```python
from build123d import *

# Parameters (mm, degrees)
SKETCH1_R                             = 14
BOSS_EXTRUDE1_DEPTH                   = 4.75
BOSS_EXTRUDE4_DEPTH                   = 7.61416499
BOSS_EXTRUDE5_START                   = 7.61416499
SKETCH5_R                             = 14
BOSS_EXTRUDE5_DEPTH                   = 7.61416499
TAP_DRILL_FOR_M4X0_7_TAP2_D           = 3.3
TAP_DRILL_FOR_M4X0_7_TAP2_DEPTH       = 13.724
TAP_DRILL_FOR_M4X0_7_TAP2_CSINK_D     = 3.35
TAP_DRILL_FOR_M4X0_7_TAP2_CSINK_ANGLE = 90
TAP_DRILL_FOR_M4X0_7_TAP2_TIP         = 0.991420021
FILLET2_R                             = 1
CBORE_FOR_M2_SHCS3_AT_2_COUNT         = 2
CBORE_FOR_M2_SHCS3_AT_2_PITCH         = 6.122934918
CBORE_FOR_M2_SHCS3_AT_3_COUNT         = 2
CBORE_FOR_M2_SHCS3_AT_3_PITCH         = 11.313708499
CBORE_FOR_M2_SHCS3_AT_4_COUNT         = 2
CBORE_FOR_M2_SHCS3_AT_4_PITCH         = 14.78207252
CBORE_FOR_M2_SHCS3_AT_5_COUNT         = 2
CBORE_FOR_M2_SHCS3_AT_5_PITCH         = 16
CBORE_FOR_M2_SHCS3_AT_6_COUNT         = 2
CBORE_FOR_M2_SHCS3_AT_6_PITCH         = 14.78207252
SKETCH20_R                            = 4
CUT_EXTRUDE2_DEPTH                    = 2.75
SKETCH21_R                            = 2
CUT_EXTRUDE3_DEPTH                    = 2.5


with BuildPart() as part:
    # Sketch1 → Boss-Extrude1 (new body)
    with BuildSketch(Plane(origin=(0, 0, 0), x_dir=(1, 0, 0), z_dir=(0, 1, 0))):
        with Locations(Location((0, 0, 0), (0, 0, 270))):
            Circle(SKETCH1_R)
    extrude(amount=-BOSS_EXTRUDE1_DEPTH)

    # Sketch4 → Boss-Extrude4 (add)
    with BuildSketch(Plane(origin=(0, 0, 0), x_dir=(1, 0, 0), z_dir=(0, 1, 0))):
        with BuildLine():
            ThreePointArc((3.9, 0), (3.062596937, 2.414642831), (0.91, 3.792347558))
            Line((0.91, 3.792347558), (-0.91, 3.792347558))
            ThreePointArc((-0.91, 3.792347558), (-2.414642831, -3.062596937), (3.9, 0))
        make_face()
        with BuildLine():
            Line((-0.91, 3.792347558), (0.91, 3.792347558))
            ThreePointArc((0.91, 3.792347558), (0, 3.9), (-0.91, 3.792347558))
        make_face()
        with BuildLine():
            Line((0.91, 3.792347558), (0.91, 4.821959978))
            Line((0.91, 4.821959978), (-0.91, 4.821959978))
            Line((-0.91, 4.821959978), (-0.91, 3.792347558))
            ThreePointArc((-0.91, 3.792347558), (0, 3.9), (0.91, 3.792347558))
        make_face()
    extrude(amount=BOSS_EXTRUDE4_DEPTH)

    # Sketch5 → Boss-Extrude5 (add)
    with BuildSketch(Plane(origin=(0, 0, 0), x_dir=(1, 0, 0), z_dir=(0, 1, 0)).offset(BOSS_EXTRUDE5_START)):
        with Locations(Location((0, 0, 0), (0, 0, 270))):
            Circle(SKETCH5_R)
        with BuildLine():
            ThreePointArc((-6.116473657, 8.411227616), (10.4, 0), (-6.116473657, -8.411227616))
            Line((-6.116473657, -8.411227616), (-6.116473657, -6.116473657))
            ThreePointArc((-6.116473657, -6.116473657), (-8.65, 0), (-6.116473657, 6.116473657))
            Line((-6.116473657, 6.116473657), (-6.116473657, 8.411227616))
        make_face(mode=Mode.SUBTRACT)
    extrude(amount=-BOSS_EXTRUDE5_DEPTH)

    # Tap Drill for M4x0.7 Tap2
    with Locations(Plane(origin=(-20, 0, 0), x_dir=(0, 0, -1), z_dir=(-1, 0, 0))):
        with Locations((0, -4.48916499)):
            CounterSinkHole(TAP_DRILL_FOR_M4X0_7_TAP2_D / 2, TAP_DRILL_FOR_M4X0_7_TAP2_CSINK_D / 2, depth=TAP_DRILL_FOR_M4X0_7_TAP2_DEPTH, counter_sink_angle=TAP_DRILL_FOR_M4X0_7_TAP2_CSINK_ANGLE)
            with Locations((0, 0, -(TAP_DRILL_FOR_M4X0_7_TAP2_DEPTH + TAP_DRILL_FOR_M4X0_7_TAP2_TIP / 2))):  # 118° drill point
                Cone(0, TAP_DRILL_FOR_M4X0_7_TAP2_D / 2, TAP_DRILL_FOR_M4X0_7_TAP2_TIP, mode=Mode.SUBTRACT)

    # Fillet2
    fillet2_edges = [part.edges().sort_by_distance(p)[0] for p in [
        (-6.116473657, 3.807082495, -8.411227616),
        (-6.116473657, 3.807082495, 8.411227616),
        (-6.116473657, 3.807082495, 6.116473657),
        (-6.116473657, 3.807082495, -6.116473657),
    ]]
    fillet(fillet2_edges, radius=FILLET2_R)

    # Sketch19 → CBORE for M2 SHCS3 (revolve, cut)
    with BuildSketch(Plane(origin=(-3.061467459, 0, -7.39103626), x_dir=(0, 0, 1), z_dir=(1, 0, 0))):
        Polygon((0, 0), (0, 5.471032743), (1.2, 4.75), (1.2, 3.5), (2.2, 3.5), (2.2, 0.025), (2.225, 0), align=None)
    cbore_for_m2_shcs3 = revolve(axis=Axis((-3.061467459, 6.35, -7.39103626), (0, -1, 0)), mode=Mode.SUBTRACT)

    # CBORE for M2 SHCS3 at 2: CBORE for M2 SHCS3 ×2
    with Locations(*[(i * CBORE_FOR_M2_SHCS3_AT_2_PITCH, 0, 0) for i in range(1, CBORE_FOR_M2_SHCS3_AT_2_COUNT)]):
        add(cbore_for_m2_shcs3, mode=Mode.SUBTRACT)

    # CBORE for M2 SHCS3 at 3: CBORE for M2 SHCS3 ×2
    with Locations(*[Vector(0.9238795325112845, 0, 0.38268343236509533) * (i * CBORE_FOR_M2_SHCS3_AT_3_PITCH) for i in range(1, CBORE_FOR_M2_SHCS3_AT_3_COUNT)]):
        add(cbore_for_m2_shcs3, mode=Mode.SUBTRACT)

    # CBORE for M2 SHCS3 at 4: CBORE for M2 SHCS3 ×2
    with Locations(*[Vector(0.7071067811865439, 0, 0.7071067811865512) * (i * CBORE_FOR_M2_SHCS3_AT_4_PITCH) for i in range(1, CBORE_FOR_M2_SHCS3_AT_4_COUNT)]):
        add(cbore_for_m2_shcs3, mode=Mode.SUBTRACT)

    # CBORE for M2 SHCS3 at 5: CBORE for M2 SHCS3 ×2
    with Locations(*[Vector(0.3826834323650841, 0, 0.9238795325112892) * (i * CBORE_FOR_M2_SHCS3_AT_5_PITCH) for i in range(1, CBORE_FOR_M2_SHCS3_AT_5_COUNT)]):
        add(cbore_for_m2_shcs3, mode=Mode.SUBTRACT)

    # CBORE for M2 SHCS3 at 6: CBORE for M2 SHCS3 ×2
    with Locations(*[(0, 0, i * CBORE_FOR_M2_SHCS3_AT_6_PITCH) for i in range(1, CBORE_FOR_M2_SHCS3_AT_6_COUNT)]):
        add(cbore_for_m2_shcs3, mode=Mode.SUBTRACT)

    # Sketch20 → Cut-Extrude2 (cut)
    with BuildSketch(Plane.XZ.offset(4.75)):
        with Locations(Location((0, 0, 0), (0, 0, 270))):
            Circle(SKETCH20_R)
    extrude(amount=-CUT_EXTRUDE2_DEPTH, mode=Mode.SUBTRACT)

    # Sketch21 → Cut-Extrude3 (cut)
    with BuildSketch(Plane(origin=(0, -2, 0), x_dir=(-1, 0, 0), z_dir=(0, -1, 0))):
        with Locations(Location((0, 0, 0), (0, 0, 90))):
            Circle(SKETCH21_R)
    extrude(amount=-CUT_EXTRUDE3_DEPTH, mode=Mode.SUBTRACT)


solid = part.part
```
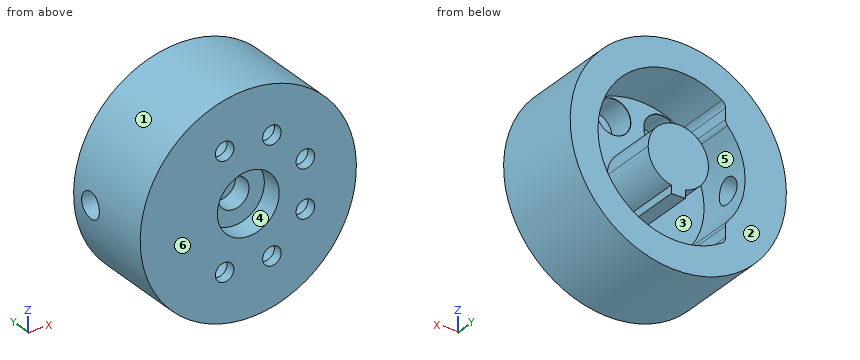
Can you work these out from the model? Positions are in its coordinate system, mm. Face numbers are marked on the shaded views. A direction names the side the tool comes from. Coordinates: 2 decimals unless noted, no trailing zeros. Write each loop counter-clockwise with the first axis right and the second up, starting at its lowest first coordinate (ties: lowest second). Pieces come first, ordered by that corner, then holes. Notation, with made-up numbers: (86.5, -35) - (101.5, -35) arc R26 cw to (101.5, -15) - close; hole circle Ø6 at (35, 14.25). An arc over 180 degrees is marked (long way). Return JSON: item names as keys, results as strings.
Q1. If we section it at B-B (z = 0.5): Please give me the cut outline in (x, y).
Computed values:
{"outline": "(-13.99, -4.75) - (-3.97, -4.75) - (-3.97, -2) - (-1.94, -2) - (-1.94, 0.5) - (1.94, 0.5) - (1.94, -2) - (3.97, -2) - (3.97, -4.75) - (13.99, -4.75) - (13.99, 7.61) - (10.39, 7.61) - (10.39, 0) - (3.87, 0) - (3.87, 7.61) - (-3.87, 7.61) - (-3.87, 0) - (-8.64, 0) - (-8.64, 2.92) - (-13.99, 2.92) - close; (-13.99, 6.06) - (-8.64, 6.06) - (-8.64, 7.61) - (-13.99, 7.61) - close"}
Q2. Thinking about a two-plate mould opening in X: for the marked faces 1, 2 and 3, which applies, +X half, -X half, draft (parallel to the pull), parting line (faces both ways), or undercut?
Computed values:
{"face 1": "parting line", "face 2": "draft", "face 3": "undercut"}
Q3. On a 3-axis mill with a long thin cutter (end or side, diameter ignored), from which of +Z, -Z, +X, -X, +Y, -Y can I reach the whole of each face in a straight line? I mean the marked faces 4, 5 and 6. Say none if no direction works.
Computed values:
{"face 4": "-Y", "face 5": "+Y", "face 6": "+Z, -Z, +X, -X, -Y"}
Q4. I'm going to push flat-ended pins straight in: pin 1 Ø3.5 at (x, z) = (2, 7.5) entering from +Y; pin 2 Ø1.5 at (x, y) = (9, -2.5) entering from +Z; pin 3 Ø7 at (x, z) = (-3.06, -7.39) entering from -Y; pin 4 Ø6.5 at (x, z) = (0, 0) entering from -Y. Where does each tip first touch, or does it pass through?
Computed values:
{"pin 1": "stops at y = 0", "pin 2": "stops at z = 11.31", "pin 3": "stops at y = -4.75", "pin 4": "stops at y = -2"}
Q5. If we section it at C-C (x = 0): Please give me the cut outline in (y, z), then the cut area to 3 significant figures.
Computed values:
{"outline": "(-4.75, -14) - (7.61, -14) - (7.61, -10.4) - (0, -10.4) - (0, -4.82) - (7.61, -4.82) - (7.61, 3.9) - (0, 3.9) - (0, 10.4) - (7.61, 10.4) - (7.61, 14) - (-4.75, 14) - (-4.75, 4) - (-2, 4) - (-2, 2) - (0.5, 2) - (0.5, -2) - (-2, -2) - (-2, -4) - (-4.75, -4) - close", "area": "222 mm2"}
Q6. If we section it at A-A (y = -1.5): Please give me the cut outline in (x, z), then the cut area to 3 significant figures.
Computed values:
{"outline": "circle Ø28 at (0, 0); hole circle Ø4.4 at (-3.06, -7.39); hole circle Ø4.4 at (-3.06, 7.39); hole circle Ø4 at (0, 0); hole circle Ø4.4 at (3.06, -7.39); hole circle Ø4.4 at (3.06, 7.39); hole circle Ø4.4 at (7.39, -3.06); hole circle Ø4.4 at (7.39, 3.06)", "area": "512 mm2"}
Q7. Please list where these lines run through material, in increasing order: L1, parallel to X at y = -2.25, z = -7.5; L2, parallel to X at y = -0.4, z = 0; L3, parallel to Y at x = 3, z = 6. Write a range as from..to.
Computed values:
{"L1": "x = -11.82..-5.26, -0.86..0.86, 5.26..11.82", "L2": "x = -14..-2, 2..14", "L3": "y = -4.75..-3.5"}
Q8. If we section it at D-D (x = -11): Please give me the cut outline in (y, z).
Computed values:
{"outline": "(-4.75, -8.66) - (7.61, -8.66) - (7.61, 8.66) - (-4.75, 8.66) - close; hole circle Ø3.3 at (4.49, 0)"}
